Part model, mm, in its own coordinate system. Face numbers are marked on the shaded views. A direction names the side the tool comes from. Give positions to 0.01 mm unless a question says otherwise; leave off trailing zeros. Order: outer loops, then holes, each group sorted by start corner. A loop starts at its lowest first (then second) coordinate and runs counter-clockwise, first axis right, second up. Notation, with made-up numbers: (33, 79.5) - (53, 79.5) arc R25 cw to (53, 110.5) - close; hole circle Ø11 at (79, 63.5). An arc over 180 degrees is marked (long way). One line per item, written item: value.
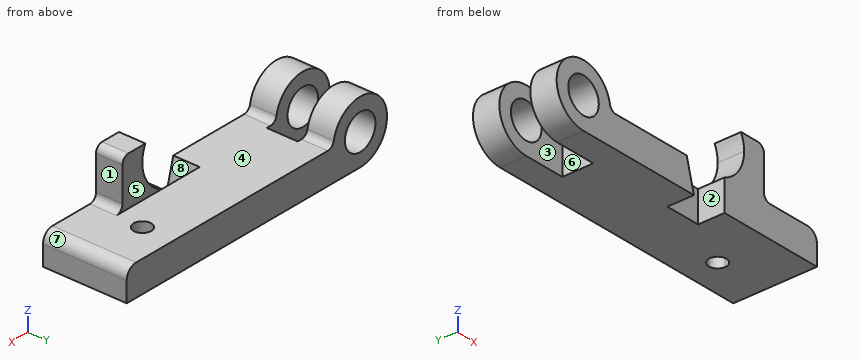
```python
from build123d import *

# Parameters (mm, degrees)
F0_R      = 12.7
F1_DEPTH  = 30.1625
F2_DEPTH  = 30.1625
F3_DEPTH  = 30.1625
F5_DEPTH  = 19.05
F6_W      = 11.1125
F6_H      = 34.798
F7_DEPTH  = 50.8
F9_DEPTH  = 50.8
F10_R     = 7.874
F11_R     = 5.08
F12_R     = 5.08
F13_R     = 5.08
F14_W     = 51.4268837869
F14_H     = 22.3266
F15_DEPTH = 50.8
F16_W     = 22.3266
F16_H     = 9.652
F16_H_2   = 12.7
F17_DEPTH = 25.4
F18_DEPTH = 50.8
F19_W     = 12.7
F19_H     = 22.3266
F20_DEPTH = 25.4
F21_W     = 4.6221852958
F21_H     = 22.3266
F22_DEPTH = 25.4


with BuildPart() as f1:
    # F0 (on Front) → F1 (new body)
    with BuildSketch(Plane.XZ):
        with BuildLine():
            Line((85.852, 0), (22.352, 0))
            ThreePointArc((22.352, 0), (-15.8052507731, 15.8052507731), (0, -22.352))
            Line((0, -22.352), (91.8464, -22.352))
            Line((91.8464, -22.352), (85.852, 0))
        make_face()
        Circle(F0_R, mode=Mode.SUBTRACT)
        with BuildLine():
            Line((99.1109187887, 0), (85.852, 0))
            Line((85.852, 0), (91.8464, -22.352))
            Line((91.8464, -22.352), (117.2464, -22.352))
            Line((117.2464, -22.352), (117.2464, 0))
            ThreePointArc((117.2464, 0), (108.1786593943, -1.6737259497), (99.1109187887, 0))
        make_face()
        with BuildLine():
            Line((117.2464, 0), (99.1109187887, 0))
            ThreePointArc((99.1109187887, 0), (108.1786593943, -1.6737259497), (117.2464, 0))
        make_face()
        Polygon((117.2464, 0), (117.2464, -22.352), (194.2084, -22.352), (194.2084, 0), (150.0886, 0), align=None)
        with BuildLine():
            ThreePointArc((133.5786593943, 23.7262740503), (129.1009036739, 9.3242014804), (117.2464, 0))
            Line((117.2464, 0), (150.0886, 0))
            Line((150.0886, 0), (150.0886, 34.798))
            Line((150.0886, 34.798), (131.0386, 34.798))
            ThreePointArc((131.0386, 34.798), (132.9355017958, 29.4059531176), (133.5786593943, 23.7262740503))
        make_face()
    extrude(amount=F1_DEPTH)

    # F0 (on Front) → F2 (join)
    with BuildSketch(Plane.XZ):
        Polygon((117.2464, 0), (117.2464, -22.352), (194.2084, -22.352), (194.2084, 0), (150.0886, 0), align=None)
    extrude(amount=-F2_DEPTH)

    # F3 (add): a face of the model
    f3_faces = [f1.faces().sort_by_distance(p)[0] for p in [
        (45.5494625665, 0, -7.7681891644),
    ]]
    extrude(f3_faces, amount=F3_DEPTH)

    # F4 (on face) → F5 (cut)
    with BuildSketch(Plane.XZ.offset(30.1625)):
        Polygon((85.852, 0), (91.8464, -22.352), (117.2464, -22.352), (117.2464, 0), align=None)
    extrude(amount=-F5_DEPTH, mode=Mode.SUBTRACT)

    # F6 (on face) → F7 (cut)
    with BuildSketch(Plane.YZ.offset(150.0886)):
        with Locations((-5.55625, 17.399)):
            Rectangle(F6_W, F6_H)
    extrude(amount=-F7_DEPTH, mode=Mode.SUBTRACT)

    # F8 (on face) → F9 (cut)
    with BuildSketch(Plane.XY):
        with BuildLine():
            ThreePointArc((161.6964, 7.8105), (159.8365280605, 12.3006280605), (155.3464, 14.1605))
            ThreePointArc((155.3464, 14.1605), (150.8562719395, 3.3203719395), (161.6964, 7.8105))
        make_face()
    extrude(amount=-F9_DEPTH, mode=Mode.SUBTRACT)

    # F10
    f10_edges = [f1.edges().sort_by_distance(p)[0] for p in [
        (194.2084, 0, 0),
    ]]
    fillet(f10_edges, radius=F10_R)

    # F11
    f11_edges = [f1.edges().sort_by_distance(p)[0] for p in [
        (150.0886, -20.6375, 34.798),
    ]]
    fillet(f11_edges, radius=F11_R)

    # F12
    f12_edges = [f1.edges().sort_by_distance(p)[0] for p in [
        (22.352, 0, 0),
    ]]
    fillet(f12_edges, radius=F12_R)

    # F13
    f13_edges = [f1.edges().sort_by_distance(p)[0] for p in [
        (150.0886, -20.6375, 0),
    ]]
    fillet(f13_edges, radius=F13_R)

    # F14 (on face) → F15 (cut)
    with BuildSketch(Plane(origin=(0, 0, -22.352), x_dir=(1, 0, 0), z_dir=(0, 0, -1))):
        with Locations((-25.7134418935, 0)):
            Rectangle(F14_W, F14_H)
    extrude(amount=-F15_DEPTH, mode=Mode.SUBTRACT)

    # F16 (on face) → F17 (cut)
    with BuildSketch(Plane(origin=(0, 0, 0), x_dir=(0, -1, 0), z_dir=(-1, 0, 0))):
        with Locations((0, 17.526)):
            Rectangle(F16_W, F16_H)
        with Locations((0, 6.35)):
            Rectangle(F16_W, F16_H_2)
    extrude(amount=-F17_DEPTH, mode=Mode.SUBTRACT)

    # F18 (cut): a face of the model
    f18_faces = [f1.faces().sort_by_distance(p)[0] for p in [
        (19.05, 0, 0),
    ]]
    extrude(f18_faces, amount=-F18_DEPTH, mode=Mode.SUBTRACT)

    # F19 (on face) → F20 (cut)
    with BuildSketch(Plane(origin=(0, 0, -22.352), x_dir=(1, 0, 0), z_dir=(0, 0, -1))):
        with Locations((6.35, 0)):
            Rectangle(F19_W, F19_H)
    extrude(amount=-F20_DEPTH, mode=Mode.SUBTRACT)

    # F21 (on face) → F22 (cut)
    with BuildSketch(Plane(origin=(0, 0, -22.352), x_dir=(1, 0, 0), z_dir=(0, 0, -1))):
        with Locations((27.7110926479, 0)):
            Rectangle(F21_W, F21_H)
    extrude(amount=-F22_DEPTH, mode=Mode.SUBTRACT)


solid = f1.part
```
1) Cut at C-C, the plane z = -3. Give the cut face in (x, y).
Outcome:
outline: (-22.15, -30.16) - (-12.34, -30.16) - (-12.34, -11.16) - (-22.15, -11.16) - close; (-22.15, 11.16) - (-12.34, 11.16) - (-12.34, 30.16) - (-22.15, 30.16) - close; (12.34, -30.16) - (86.66, -30.16) - (86.66, -11.11) - (117.25, -11.11) - (117.25, -30.16) - (192.52, -30.16) - (192.52, 30.16) - (12.34, 30.16) - (12.34, 11.16) - (30.02, 11.16) - (30.02, -11.16) - (12.34, -11.16) - close; hole circle Ø12.7 at (155.35, 7.81)
2) Cut at D-D, the plane x = 7. Give the cut face in (y, z).
Outcome:
outline: (-30.16, -22.35) - (-11.16, -22.35) - (-11.16, -10.6) - (-30.16, -10.6) - close; (-30.16, 10.6) - (-11.16, 10.6) - (-11.16, 21.23) - (-30.16, 21.23) - close; (11.16, -22.35) - (30.16, -22.35) - (30.16, -10.6) - (11.16, -10.6) - close; (11.16, 10.6) - (30.16, 10.6) - (30.16, 21.23) - (11.16, 21.23) - close
3) Cut at A-A, the plane y = -16. Give the cut face in (x, z).
Outcome:
outline: (0, -22.35) - (91.85, -22.35) - (85.85, 0) - (26.96, 0) arc R5.08 cw to (21.97, 4.14) arc R22.35 ccw (long way) to start; (117.25, -22.35) - (194.21, -22.35) - (194.21, -7.87) arc R7.87 ccw to (186.33, 0) - (155.17, 0) arc R5.08 cw to (150.09, 5.08) - (150.09, 29.72) arc R5.08 ccw to (145.01, 34.8) - (131.04, 34.8) arc R25.4 cw to (117.25, 0) - close; hole circle Ø25.4 at (0, 0)
4) Mould opens along X. For the marked faces 5, 6, 7 and 8 say: released by +X, released by -X, zero draft, split by the parting line, or undercut.
Outcome:
face 5: zero draft
face 6: released by -X
face 7: released by +X
face 8: undercut
5) Cut at B-B, the plane x = 153. Give the cut face in (y, z).
Outcome:
outline: (-30.16, -22.35) - (1.91, -22.35) - (1.91, 0) - (-11.11, 0) - (-11.11, 0.49) - (-30.16, 0.49) - close; (13.71, -22.35) - (30.16, -22.35) - (30.16, 0) - (13.71, 0) - close
6) Drill centre lines: line 1 along Z through (x, y) = (0, -19); line 2 along Y through (x, z) = (14, -13.5); line 3 along Z through (x, y) = (82, -26.5). Where is each one in solid material? Low to high. Write a range as from..to.
Outcome:
line 1: z = -22.35..-12.7, 12.7..22.35
line 2: y = -30.16..-11.16, 11.16..30.16
line 3: z = -22.35..0
7) Which spindle directions (+Z, -Z, +X, -X, +Y, -Y) get a long thin tool onto all of the face, cutting with end or side? Do the marked faces 1, 2, 3 and 4. Say none if no direction does.
Outcome:
face 1: +Z, +X, +Y, -Y
face 2: +Z, -Z, -Y
face 3: +Z, -Z, -X
face 4: +Z, +Y
8) Pin check, flat tips, straight feed: pin 1 (20.5 mm diameter, centred on x = 0, z = 0, fed in from -Y); pin 2 (16.5 mm diameter, centred on x = 155.35, y = 7.81, fed in from +Z); pin 3 (24.5 mm diameter, centred on x = 99.5, z = -7.5, fed in from -Y); pin 4 (11 mm diameter, centred on y = -0.5, z = -15.5, fed in from -X). Stop position of each tip, or through.
Outcome:
pin 1: passes through
pin 2: stops at z = 0
pin 3: stops at y = -30.16
pin 4: stops at x = 30.02
